from build123d import *

# Parameters (mm, degrees)
SKETCH3_R               = 2.15
BOSS_EXTRUDE1_DEPTH     = 1524
CIRPATTERN1_COUNT       = 2
CUT_EXTRUDE1_DEPTH      = 10
CUT_EXTRUDE1_DEPTH_BACK = 23
SKETCH4_OUTSIDE_W       = 3659.666
SKETCH4_OUTSIDE_H       = 651.666
SKETCH4_OUTSIDE_W_2     = 600
SKETCH4_OUTSIDE_H_2     = 40


with BuildPart() as part:
    # Sketch3 → Boss-Extrude1 (new, symmetric)
    with BuildSketch(Plane.XY):
        with BuildLine():
            Line((-8.30911066, 7.475083014), (-9.008684239, 7.499512662))
            ThreePointArc((-9.008684239, 7.499512662), (-9.582202525, 7.285082961), (-9.836116498, 6.727919597))
            Line((-9.836116498, 6.727919597), (-9.986803685, 2.412803152))
            ThreePointArc((-9.986803685, 2.412803152), (-9.995837451, 2.069746735), (-9.99898368, 1.726585818))
            Line((-9.99898368, 1.726585818), (-10, 0))
            Line((-10, 0), (-7.916458339, 0))
            ThreePointArc((-7.916458339, 0), (-7.764217404, 0.765366865), (-7.330671901, 1.414213562))
            Line((-7.330671901, 1.414213562), (-3.22356512, 5.521320344))
            ThreePointArc((-3.22356512, 5.521320344), (-2.250295073, 6.171638598), (-1.102244776, 6.4))
            Line((-1.102244776, 6.4), (1.102244776, 6.4))
            ThreePointArc((1.102244776, 6.4), (2.250295073, 6.171638598), (3.22356512, 5.521320344))
            Line((3.22356512, 5.521320344), (7.330671901, 1.414213562))
            ThreePointArc((7.330671901, 1.414213562), (7.764217404, 0.765366865), (7.916458339, 0))
            Line((7.916458339, 0), (10, 0))
            Line((10, 0), (9.99898368, 1.726585818))
            ThreePointArc((9.99898368, 1.726585818), (9.995837451, 2.069746735), (9.986803685, 2.412803152))
            Line((9.986803685, 2.412803152), (9.836116498, 6.727919597))
            ThreePointArc((9.836116498, 6.727919597), (9.582202525, 7.285082961), (9.008684239, 7.499512662))
            Line((9.008684239, 7.499512662), (8.30911066, 7.475083014))
            ThreePointArc((8.30911066, 7.475083014), (8.100174399, 7.379865274), (8.019763261, 7.164795917))
            Line((8.019763261, 7.164795917), (8.093719461, 5.046967452))
            ThreePointArc((8.093719461, 5.046967452), (7.631170264, 4.313871343), (6.779559917, 4.47555462))
            Line((6.779559917, 4.47555462), (4.478679656, 6.77643488))
            ThreePointArc((4.478679656, 6.77643488), (3.828361402, 7.749704927), (3.6, 8.897755224))
            Line((3.6, 8.897755224), (3.6, 11.102244776))
            ThreePointArc((3.6, 11.102244776), (3.828361402, 12.250295073), (4.478679656, 13.22356512))
            Line((4.478679656, 13.22356512), (6.779559917, 15.52444538))
            ThreePointArc((6.779559917, 15.52444538), (7.631170264, 15.686128657), (8.093719461, 14.953032548))
            Line((8.093719461, 14.953032548), (8.019763261, 12.835204083))
            ThreePointArc((8.019763261, 12.835204083), (8.100174399, 12.620134726), (8.30911066, 12.524916986))
            Line((8.30911066, 12.524916986), (9.008684239, 12.500487338))
            ThreePointArc((9.008684239, 12.500487338), (9.582202525, 12.714917039), (9.836116498, 13.272080403))
            Line((9.836116498, 13.272080403), (9.998781654, 17.930201007))
            ThreePointArc((9.998781654, 17.930201007), (9.414213562, 19.414213562), (7.930201007, 19.998781654))
            Line((7.930201007, 19.998781654), (3.272080403, 19.836116498))
            ThreePointArc((3.272080403, 19.836116498), (2.714917039, 19.582202525), (2.500487338, 19.008684239))
            Line((2.500487338, 19.008684239), (2.524916986, 18.30911066))
            ThreePointArc((2.524916986, 18.30911066), (2.620134726, 18.100174399), (2.835204083, 18.019763261))
            Line((2.835204083, 18.019763261), (4.953032548, 18.093719461))
            ThreePointArc((4.953032548, 18.093719461), (5.686128657, 17.631170264), (5.52444538, 16.779559917))
            Line((5.52444538, 16.779559917), (3.22356512, 14.478679656))
            ThreePointArc((3.22356512, 14.478679656), (2.250295073, 13.828361402), (1.102244776, 13.6))
            Line((1.102244776, 13.6), (-1.102244776, 13.6))
            ThreePointArc((-1.102244776, 13.6), (-2.250295073, 13.828361402), (-3.22356512, 14.478679656))
            Line((-3.22356512, 14.478679656), (-5.52444538, 16.779559917))
            ThreePointArc((-5.52444538, 16.779559917), (-5.686128657, 17.631170264), (-4.953032548, 18.093719461))
            Line((-4.953032548, 18.093719461), (-2.835204083, 18.019763261))
            ThreePointArc((-2.835204083, 18.019763261), (-2.620134726, 18.100174399), (-2.524916986, 18.30911066))
            Line((-2.524916986, 18.30911066), (-2.500487338, 19.008684239))
            ThreePointArc((-2.500487338, 19.008684239), (-2.714917039, 19.582202525), (-3.272080403, 19.836116498))
            Line((-3.272080403, 19.836116498), (-7.930201007, 19.998781654))
            ThreePointArc((-7.930201007, 19.998781654), (-9.414213562, 19.414213562), (-9.998781654, 17.930201007))
            Line((-9.998781654, 17.930201007), (-9.836116498, 13.272080403))
            ThreePointArc((-9.836116498, 13.272080403), (-9.582202525, 12.714917039), (-9.008684239, 12.500487338))
            Line((-9.008684239, 12.500487338), (-8.30911066, 12.524916986))
            ThreePointArc((-8.30911066, 12.524916986), (-8.100174399, 12.620134726), (-8.019763261, 12.835204083))
            Line((-8.019763261, 12.835204083), (-8.093719461, 14.953032548))
            ThreePointArc((-8.093719461, 14.953032548), (-7.631170264, 15.686128657), (-6.779559917, 15.52444538))
            Line((-6.779559917, 15.52444538), (-4.478679656, 13.22356512))
            ThreePointArc((-4.478679656, 13.22356512), (-3.828361402, 12.250295073), (-3.6, 11.102244776))
            Line((-3.6, 11.102244776), (-3.6, 8.897755224))
            ThreePointArc((-3.6, 8.897755224), (-3.828361402, 7.749704927), (-4.478679656, 6.77643488))
            Line((-4.478679656, 6.77643488), (-6.779559917, 4.47555462))
            ThreePointArc((-6.779559917, 4.47555462), (-7.631170264, 4.313871343), (-8.093719461, 5.046967452))
            Line((-8.093719461, 5.046967452), (-8.019763261, 7.164795917))
            ThreePointArc((-8.019763261, 7.164795917), (-8.100174399, 7.379865274), (-8.30911066, 7.475083014))
        make_face()
        with Locations((0, 10)):
            Circle(SKETCH3_R, mode=Mode.SUBTRACT)
    boss_extrude1 = extrude(amount=BOSS_EXTRUDE1_DEPTH, both=True)

    # CirPattern1: Boss-Extrude1 ×2 about axis
    cirpattern1_axis = Axis((0, 0, 0), (0, 0, 1))
    for i in range(1, CIRPATTERN1_COUNT):
        add(boss_extrude1.rotate(cirpattern1_axis, i * 360 / CIRPATTERN1_COUNT))

    # Sketch4 outside → Cut-Extrude1 (cut, two sides: drawn at the far end of the back side and taken through both)
    with BuildSketch(Plane(origin=(3.6, 0, 0), x_dir=(0, 0, -1), z_dir=(1, 0, 0)).offset(-CUT_EXTRUDE1_DEPTH_BACK)):
        Rectangle(SKETCH4_OUTSIDE_W, SKETCH4_OUTSIDE_H)
        with Locations((-1224, 0)):
            Rectangle(SKETCH4_OUTSIDE_W_2, SKETCH4_OUTSIDE_H_2, mode=Mode.SUBTRACT)
    extrude(amount=CUT_EXTRUDE1_DEPTH + CUT_EXTRUDE1_DEPTH_BACK, mode=Mode.SUBTRACT)


solid = part.part
Geometry check sheet. Reference: the model listing, model coordinates, mm. Round coordinates to 2 decimals unless told otherwise and drop trailing zeros. Use one line per item in the form item = value.
1. Cross-section at A-A, the plane z = 1321.5. Count the separate pieces of the cut face and the enclosed holes in it, plus the area to 3 significant figures.
Working result:
separate_pieces = 1
enclosed_holes = 3
area = 327 mm^2
2. Go/stop test with flat-tipped pins: pin 1 (0.7 mm diameter, centred on y = 9.5, z = 1293.5, fed in from -X); pin 2 (1 mm diameter, centred on x = 6, z = 1021.5, fed in from +Y); pin 3 (4 mm diameter, centred on y = 5, z = 1053.5, fed in from +X); pin 4 (4 mm diameter, centred on x = 0, y = -10, fed in from -Z). Record where each tip stops, or that it passes through.
Working result:
pin_1 = -3.6
pin_2 = 19.95
pin_3 = 9.97
pin_4 = through
3. Scan lines: line 1 along X through (y, z) = (7, 1164.5); line 2 along Y through (x, z) = (0, 1238); line 3 along X through (y, z) = (-5.5, 952.5). Record each from-to range of solid material in increasing order. Write a range as from..to.
Working result:
line_1 = -9.78..-8.03, -4.28..4.28, 8.03..9.78
line_2 = -13.6..-12.15, -7.85..-6.4, 6.4..7.85, 12.15..13.6
line_3 = -9.88..-8.08, -5.76..-3.24, 3.24..5.76, 8.08..9.88
4. Mould release check, pull along Z, two halves, no side actions. Record for faces 1 (the face through (4, -5, 924)), 2 (the face through (-4, -5, 1524)): pulls with the +Z half, pulls with the -Z half, needs draft (parallel to the pull), parting line crosses it, or undercut.
Working result:
face_1 = pulls with the -Z half
face_2 = pulls with the +Z half
